```python
from build123d import *

# Parameters (mm, degrees)
F0_W        = 206.1633169651
F0_H        = 136.7557346821
F3_DEPTH    = 38.1348449737
F7_T1_DEPTH = 998.2832658749
F8_W        = 206.1633169651
F8_H        = 136.7557346821
F8_W_2      = 174.7721135616
F8_H_2      = 16.5176689625
F8_W_3      = 117.4946576357
F8_H_3      = 18.816370517
F2_W        = 206.1633169651
F2_H        = 136.7557346821
F9_DEPTH    = 121.7797268182


# Not quite as in the source:
# - a fillet or chamfer that OpenCascade refuses, or shapes differently, is made with other operations: its cross-section is extruded or revolved along the edge and cut away or added
# - the program builds the solid bodies; features that only make, move or delete a surface that nothing else refers to are left out


with BuildPart() as f3:
    # F0 (on Front) → F3 (new body)
    with BuildSketch(Plane.XZ):
        with Locations((1.0583624244, 0.0938400626)):
            Rectangle(F0_W, F0_H)
    extrude(amount=F3_DEPTH)

    # F7: fillet of radius 203.2 on 2 edges, made by hand

    # F7_s2 → F7_t1 (cut)
    with BuildSketch(Plane.XZ.offset(-480.0742104506)):
        with BuildLine():
            ThreePointArc((104.1400209069, -68.2840272784), (29.9847726477, 30.7886471902), (-87.8896632733, 68.4717074037))
            Line((-87.8896632733, 68.4717074037), (104.1400209069, 68.4717074037))
            Line((104.1400209069, 68.4717074037), (104.1400209069, -68.2840272784))
        make_face()
        with BuildLine():
            ThreePointArc((90.0063881221, 68.4717074037), (-27.868047799, 30.7886471902), (-102.0232960582, -68.2840272784))
            Line((-102.0232960582, -68.2840272784), (-102.0232960582, 68.4717074037))
            Line((-102.0232960582, 68.4717074037), (90.0063881221, 68.4717074037))
        make_face()
    extrude(amount=F7_T1_DEPTH, mode=Mode.SUBTRACT)

    # F8 (on face) + F2 (on face) → F9 (join)
    with BuildSketch(Plane.XZ):
        with Locations((1.0583624244, 0.0938400626)):
            Rectangle(F8_W, F8_H)
        with Locations((0, -32.6089076698)):
            Rectangle(F8_W_2, F8_H_2, mode=Mode.SUBTRACT)
        with Locations((10.9684318304, -3.3599911258)):
            Rectangle(F8_W_3, F8_H_3, mode=Mode.SUBTRACT)
    with BuildSketch(Plane.XZ):
        with Locations((1.0583624244, 0.0938400626)):
            Rectangle(F2_W, F2_H)
    extrude(amount=-F9_DEPTH)


solid = f3.part
```
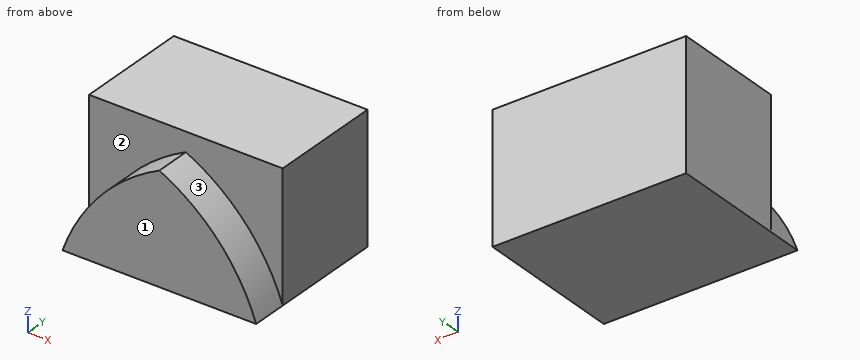
Input: part model. Units: mm. Frame: model coordinates. Face numbers are marked on the shaded views. A direction names the side the tool comes from. Round coordinates to 2 decimals unless told otherwise and drop trailing zeros. Loops run counter-clockwise (first coordinate to the right, second up) from the corner with the lowest first, then second, coordinate; pieces in that order, holes last.
1) Section query A-A on z = -5.5. Return the cut outline in (x, y), plus the area to 3 significant figures.
Ans:
outline: (-102.02, 0) - (-66.81, 0) - (-66.81, -38.13) - (68.92, -38.13) - (68.92, 0) - (104.14, 0) - (104.14, 121.78) - (-102.02, 121.78) - close
area: 30,300 mm2
2) Set-up query: the marked faces 1, 2 and 3. Return all of +Z, -Z, +X, -X, +Y, -Y with unobstructed straight access to the full face (end or side cutting, diameter ignored); none if empty.
Ans:
face 1: +Z, -Z, +X, -X, -Y
face 2: +Z, -Y
face 3: +Z, +X, -Y
3) Pin query (flat end, axial travel): pin 1 (4 mm diameter, centred on y = -13, z = -26, fed in from -X); pin 2 (6 mm diameter, centred on y = -7, z = 11, fed in from -X). Return the tip coordinate at first contact, or that it passes through.
Ans:
pin 1: stops at x = -82.91
pin 2: stops at x = -54.63
4) Material intervals for line 1 (Y direction, x = -93, z = 42.5); line 2 (X direction, y = -4.5, z = 23.5); line 3 (Z direction, x = 33, y = -8.5), sorted ascending.
Ans:
line 1: y = 0 to 121.78
line 2: x = -37.48 to 39.6
line 3: z = -68.28 to 28.6
5) Section query B-B on y = -7. Return the cut outline in (x, z), plus the area to 3 significant figures.
Ans:
outline: (-102.02, -68.28) - (104.14, -68.28) arc R203.2 ccw to (1.06, 47.97) arc R203.2 ccw to start
area: 15,200 mm2
6) Section query C-C on x = 37.5. Return the cut outline in (y, z), plus the area to 3 significant figures.
Ans:
outline: (-38.13, -68.28) - (121.78, -68.28) - (121.78, 68.47) - (0, 68.47) - (0, 25.17) - (-38.13, 25.17) - close
area: 20,200 mm2
7) Section query D-D on z = 54. Return the cut outline in (x, y).
Ans:
outline: (-102.02, 0) - (104.14, 0) - (104.14, 121.78) - (-102.02, 121.78) - close
